Model file for the job. Use its own axes, mm. Give positions to 0.01 mm unless a question says otherwise; leave off trailing zeros. Loops run counter-clockwise (first coordinate to the right, second up) from the corner with the lowest first, then second, coordinate; pieces in that order, holes last. Notation, with made-up numbers: M -11,79.25 L 27,79.25 A17 cw 27,96.25 Z; hole C 3.25,1 d6. An arc over 180 degrees is marked long. Use CSV: the item, a comma, the result in double quotes. Start each with the question number.
(1) Slice it at C-C on x = 13.5. List the corners of the cut face in (y, z), and give its area (3 significant figures).
(2) Slice it at B-B on z = 27.5. List the corners of the cut face in (x, y), and give its area (3 significant figures).
(3) Wall check: line 1 along Z through (x, y) = (7.5, -18); line 2 along X through (y, z) = (-8.5, 13) (3 decimals); line 3 along X through (y, z) = (-23.5, 35). Give the ranges that are in metal, low to high. Write a range as from..to.
(4) Flat gauge pins, fed straight in: P1, Ø5, axis at y = -21.5, z = 14.5, coming from the -X side; P2, Ø1.5, axis at x = 12, y = -21, coming from the +Z side; P3, Ø10, axis at x = 12.5, y = -14, coming from the -Z side. Where does each tip first touch, or does it go through?
```python
from build123d import *

# Parameters (mm, degrees)
F0_W     = 80
F0_H     = 40
F1_DEPTH = 25
F2_R     = 20
F3_R     = 19.99999
F4_R     = 5


# Not quite as in the source:
# - a fillet or chamfer is up to 0.001 mm smaller than in the source, because OpenCascade refuses the exact size


with BuildPart() as f1:
    # F0 (on Front) → F1 (new body)
    with BuildSketch(Plane.XZ):
        with Locations((40, 20)):
            Rectangle(F0_W, F0_H)
    extrude(amount=F1_DEPTH)

    # F2
    f2_edges = [f1.edges().sort_by_distance(p)[0] for p in [
        (0, -12.5, 40),
    ]]
    fillet(f2_edges, radius=F2_R)

    # F3 (radius 20 in the source; OpenCascade refuses exactly that, so slightly less here)
    f3_edges = [f1.edges().sort_by_distance(p)[0] for p in [
        (0, -12.5, 0),
    ]]
    fillet(f3_edges, radius=F3_R)

    # F4
    f4_edges = [f1.edges().sort_by_distance(p)[0] for p in [
        (80, -12.5, 40),
        (80, -12.5, 0),
    ]]
    fillet(f4_edges, radius=F4_R)


solid = f1.part
```
Reply:
1,outline,"M -25,1.09 L 0,1.09 L 0,38.91 L -25,38.91 Z"
1,area,"946 mm^2"
2,outline,"M 1.46,-25 L 80,-25 L 80,0 L 1.46,0 Z"
2,area,"1,960 mm^2"
3,line 1,"z = 4.39..35.61"
3,line 2,"x = 1.265..80"
3,line 3,"x = 6.77..80"
4,P1,"stops at x = 0.23"
4,P2,"stops at z = 38.64"
4,P3,"stops at z = 0.16"
